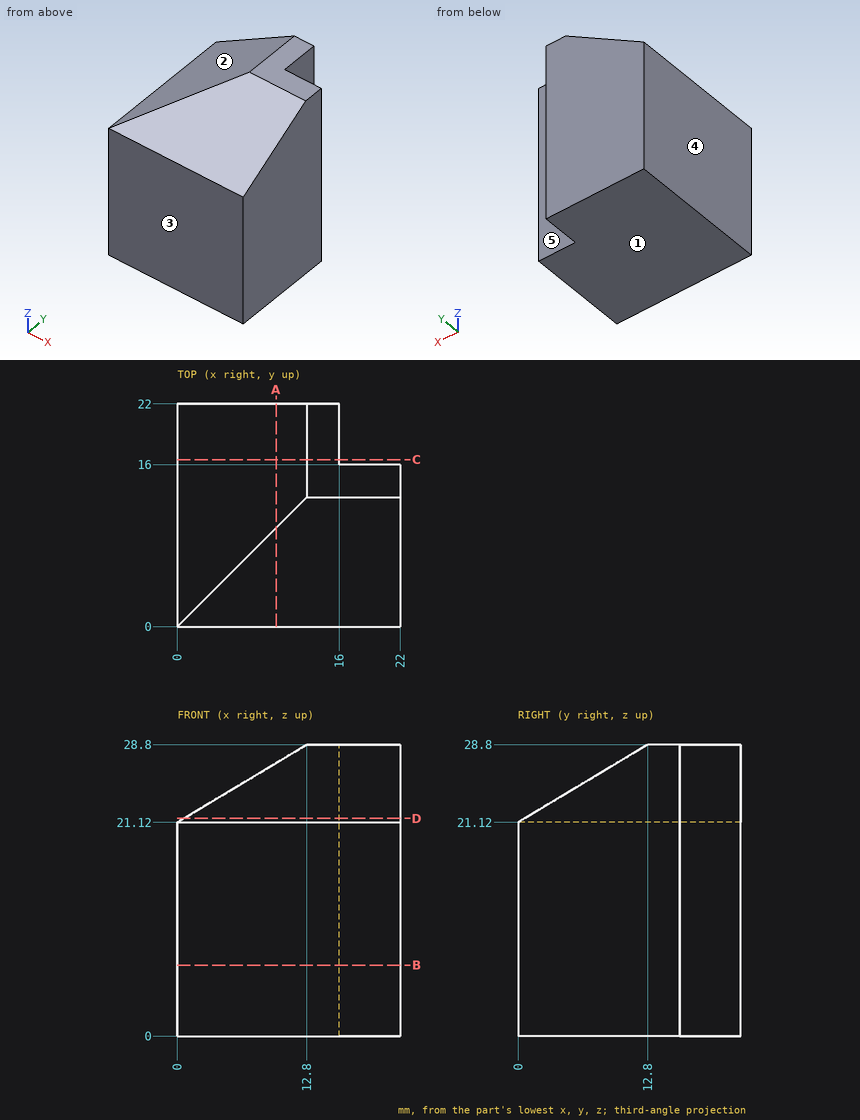
Can you work these out from the drawing? Everything is in mm from the part's minimum corner. A direction names the side the tool comes from. Give positions to 0.01 mm unless a question says otherwise; leave off trailing zeros. Order: outer loops, then holes, each group sorted by start corner. A loop starts at its lowest first (then second) coordinate and runs counter-clockwise, first axis right, second up.
1. Suppose I cut it at C-C (y = 16.5). List the corners of the cut face in (x, z) for me.
2. Suppose I cut it at D-D (z = 21.5). List the corners of the cut face in (x, y) for me, plus the area to 3 significant figures.
3. Suppose I cut it at A-A (x = 9.75). List the corners of the cut face in (y, z) for me.
4. Suppose I cut it at B-B (z = 7). List the corners of the cut face in (x, y) for me, plus the area to 3 significant figures.
5. For the marked faces 4 and 5, which set-ups out of +Z, -Z, +X, -X, +Y, -Y let a thin tool reach every point of the face, with its end or its side?
6. I need wall thicknesses on L1, parallel to Y at x = 17.75, z = 2.25; L2, parallel to X at y = 19.25, z = 24.75. Which ranges of each line are inside material? Lowest first, please.
7. Will these pins go through, and if not, where does the flat tip stop? P1, Ø1, axis at x = 17, y = 8.5, coming from the +Z side; P2, Ø3, axis at y = 3.5, z = 13.5, coming from the -X side; P3, Ø6, axis at x = 18, y = 3.5, coming from the +Z side; P4, Ø2, axis at y = 3, z = 23.5, coming from the -X side.
8. We'd pull the mould along Z, two halves only. Please class the marked faces 1, 2 and 3: pulls with the +Z half, pulls with the -Z half, needs draft (parallel to the pull), parting line crosses it, or undercut.
Solved:
1. outline: (0, 0) - (16, 0) - (16, 28.8) - (12.8, 28.8) - (0, 21.12) - close
2. outline: (0.63, 0.63) - (22, 0.63) - (22, 16) - (16, 16) - (16, 22) - (0.63, 22) - close
2. area: 421 mm2
3. outline: (0, 0) - (22, 0) - (22, 26.97) - (9.75, 26.97) - (0, 21.12) - close
4. outline: (0, 0) - (22, 0) - (22, 16) - (16, 16) - (16, 22) - (0, 22) - close
4. area: 448 mm2
5. face 4: +Z, -Z, -X, +Y, -Y
5. face 5: +Z, -Z, +X, +Y
6. L1: y = 0 to 16
6. L2: x = 6.05 to 16
7. P1: stops at z = 26.52
7. P2: stops at x = 0
7. P3: stops at z = 25.02
7. P4: stops at x = 2.3
8. face 1: pulls with the -Z half
8. face 2: pulls with the +Z half
8. face 3: needs draft
